Read the model definition and answer for the solid it produces. Units are mm, in the model's axes. A direction names the side the tool comes from. Coordinates: 2 decimals unless noted, no trailing zeros.
Item 1: A tool of negligible diameter and unlimited length cuts with its end or side. For faces 1 (the face through (3.035, 15.486, 2.465)), 2 (the face through (-3.035, -15.486, 2.465)), 3 (the face through (-2, 9, 5)), 4 (the face through (-1.5, 11.4, -1)), from which of +Z, -Z, +X, -X, +Y, -Y can it reach the whole face along a straight path? Write none if from no direction.
Item 2: Each of these flat-tipped pins is pushed along its axis until it touches: P1, Ø1.5, axis at x = 2, z = 1.5, coming from the +Y side; P2, Ø20.5, axis at x = 0, y = 0, coming from the +Z side; P3, Ø5, axis at y = 8, z = 3.5, coming from the +X side; P4, Ø11.5, axis at x = -0.5, y = 2, coming from the -Z side. Where does it stop, or does it pass through?
Item 3: Straight lines are drawn through the part: probe 1 along Y at (x, z) = (0, 5.75); probe 2 along Z at (x, y) = (-10.5, -10); probe 3 along X at (y, z) = (1.5, 3.25). For each, find the intervals that lie inside material, in ascending order.
Item 4: Determine the mould class of faces 5 (the face through (-13.84, 7.99, 2.46)), 6 (the face through (5.465, -15.015, 2.465)), 7 (the face through (15.736, -2.775, 2.465)), 8 (the face through (-2, 9, 0)) for opening direction Y: released by +Y, released by -Y, zero draft, split by the parting line, or undercut.
from build123d import *

# Parameters (mm, degrees)
F1_DEPTH = 5
F2_R     = 13.25
F2_R_2   = 11.5
F3_DEPTH = 2.5
F4_R     = 13.25
F4_R_2   = 11.5
F5_DEPTH = 2.5
F6_R     = 0.5


with BuildPart() as f1:
    # F0 (on Top) → F1 (new body)
    with BuildSketch(Plane.XY):
        with BuildLine():
            Line((3.0937469913, 8.5), (4.9592920782, 13.6255430014))
            ThreePointArc((4.9592920782, 13.6255430014), (2.5178985762, 14.2797124187), (0, 14.5))
            Line((0, 14.5), (0, 8.5))
            Line((0, 8.5), (3.0937469913, 8.5))
        make_face()
        with BuildLine():
            ThreePointArc((0, 14.5), (2.5178985762, 14.2797124187), (4.9592920782, 13.6255430014))
            Line((4.9592920782, 13.6255430014), (5.9853525082, 16.4446208638))
            Line((5.9853525082, 16.4446208638), (0, 14.5))
        make_face()
        with BuildLine():
            Line((-3.0937469913, 8.5), (0, 8.5))
            Line((0, 8.5), (0, 14.5))
            ThreePointArc((0, 14.5), (-2.5178985762, 14.2797124187), (-4.9592920782, 13.6255430014))
            Line((-4.9592920782, 13.6255430014), (-3.0937469913, 8.5))
        make_face()
        with BuildLine():
            ThreePointArc((-4.9592920782, 13.6255430014), (-2.5178985762, 14.2797124187), (0, 14.5))
            Line((0, 14.5), (0, 17.5))
            Line((0, 17.5), (-4.9592920782, 13.6255430014))
        make_face()
        with BuildLine():
            Line((5.8143424365, 6.9292634873), (9.3204203405, 11.1076444252))
            ThreePointArc((9.3204203405, 11.1076444252), (7.25, 12.5573683549), (4.9592920782, 13.6255430014))
            Line((4.9592920782, 13.6255430014), (3.0937469913, 8.5))
            Line((3.0937469913, 8.5), (4.9074772881, 8.5))
            Line((4.9074772881, 8.5), (5.8143424365, 6.9292634873))
        make_face()
        with BuildLine():
            ThreePointArc((4.9592920782, 13.6255430014), (7.25, 12.5573683549), (9.3204203405, 11.1076444252))
            Line((9.3204203405, 11.1076444252), (11.2487831695, 13.4057777546))
            Line((11.2487831695, 13.4057777546), (4.9592920782, 13.6255430014))
        make_face()
        with BuildLine():
            ThreePointArc((9.3204203405, 11.1076444252), (11.1076444252, 9.3204203405), (12.5573683549, 7.25))
            Line((12.5573683549, 7.25), (15.1554445662, 8.75))
            Line((15.1554445662, 8.75), (9.3204203405, 11.1076444252))
        make_face()
        with BuildLine():
            Line((8.9080894278, 1.5707365127), (14.2797124187, 2.5178985762))
            ThreePointArc((14.2797124187, 2.5178985762), (13.6255430014, 4.9592920782), (12.5573683549, 7.25))
            Line((12.5573683549, 7.25), (7.3612159322, 4.25))
            Line((7.3612159322, 4.25), (8.9080894278, 1.5707365127))
        make_face()
        with BuildLine():
            ThreePointArc((12.5573683549, 7.25), (13.6255430014, 4.9592920782), (14.2797124187, 2.5178985762))
            Line((14.2797124187, 2.5178985762), (17.2341356777, 3.0388431092))
            Line((17.2341356777, 3.0388431092), (12.5573683549, 7.25))
        make_face()
        with BuildLine():
            ThreePointArc((14.2797124187, -2.5178985762), (14.4448231223, -1.2637582698), (14.5, 0))
            ThreePointArc((14.5, 0), (14.4448231223, 1.2637582698), (14.2797124187, 2.5178985762))
            Line((14.2797124187, 2.5178985762), (8.9080894278, 1.5707365127))
            Line((8.9080894278, 1.5707365127), (9.8149545762, 0))
            Line((9.8149545762, 0), (8.9080894278, -1.5707365127))
            Line((8.9080894278, -1.5707365127), (14.2797124187, -2.5178985762))
        make_face()
        with BuildLine():
            ThreePointArc((14.2797124187, 2.5178985762), (14.4448231223, 1.2637582698), (14.5, 0))
            ThreePointArc((14.5, 0), (14.4448231223, -1.2637582698), (14.2797124187, -2.5178985762))
            Line((14.2797124187, -2.5178985762), (17.2341356777, -3.0388431092))
            Line((17.2341356777, -3.0388431092), (14.2797124187, 2.5178985762))
        make_face()
        with BuildLine():
            ThreePointArc((12.5573683549, -7.25), (13.6255430014, -4.9592920782), (14.2797124187, -2.5178985762))
            Line((14.2797124187, -2.5178985762), (8.9080894278, -1.5707365127))
            Line((8.9080894278, -1.5707365127), (7.3612159322, -4.25))
            Line((7.3612159322, -4.25), (12.5573683549, -7.25))
        make_face()
        with BuildLine():
            Line((15.1554445662, -8.75), (14.2797124187, -2.5178985762))
            ThreePointArc((14.2797124187, -2.5178985762), (13.6255430014, -4.9592920782), (12.5573683549, -7.25))
            Line((12.5573683549, -7.25), (15.1554445662, -8.75))
        make_face()
        with BuildLine():
            ThreePointArc((9.3204203405, -11.1076444252), (11.1076444252, -9.3204203405), (12.5573683549, -7.25))
            Line((12.5573683549, -7.25), (7.3612159322, -4.25))
            Line((7.3612159322, -4.25), (5.8143424365, -6.9292634873))
            Line((5.8143424365, -6.9292634873), (9.3204203405, -11.1076444252))
        make_face()
        with BuildLine():
            Line((11.2487831695, -13.4057777546), (12.5573683549, -7.25))
            ThreePointArc((12.5573683549, -7.25), (11.1076444252, -9.3204203405), (9.3204203405, -11.1076444252))
            Line((9.3204203405, -11.1076444252), (11.2487831695, -13.4057777546))
        make_face()
        with BuildLine():
            ThreePointArc((4.9592920782, -13.6255430014), (7.25, -12.5573683549), (9.3204203405, -11.1076444252))
            Line((9.3204203405, -11.1076444252), (5.8143424365, -6.9292634873))
            Line((5.8143424365, -6.9292634873), (4.9074772881, -8.5))
            Line((4.9074772881, -8.5), (3.0937469913, -8.5))
            Line((3.0937469913, -8.5), (4.9592920782, -13.6255430014))
        make_face()
        with BuildLine():
            Line((5.9853525082, -16.4446208638), (9.3204203405, -11.1076444252))
            ThreePointArc((9.3204203405, -11.1076444252), (7.25, -12.5573683549), (4.9592920782, -13.6255430014))
            Line((4.9592920782, -13.6255430014), (5.9853525082, -16.4446208638))
        make_face()
        with BuildLine():
            Line((0, -17.5), (4.9592920782, -13.6255430014))
            ThreePointArc((4.9592920782, -13.6255430014), (2.5178985762, -14.2797124187), (0, -14.5))
            Line((0, -14.5), (0, -17.5))
        make_face()
        with BuildLine():
            Line((0, -8.5), (-3.0937469913, -8.5))
            Line((-3.0937469913, -8.5), (-4.9592920782, -13.6255430014))
            ThreePointArc((-4.9592920782, -13.6255430014), (-2.5178985762, -14.2797124187), (0, -14.5))
            Line((0, -14.5), (0, -8.5))
        make_face()
        with BuildLine():
            ThreePointArc((0, -14.5), (-2.5178985762, -14.2797124187), (-4.9592920782, -13.6255430014))
            Line((-4.9592920782, -13.6255430014), (-5.9853525082, -16.4446208638))
            Line((-5.9853525082, -16.4446208638), (0, -14.5))
        make_face()
        with BuildLine():
            Line((7.3612159322, 4.25), (12.5573683549, 7.25))
            ThreePointArc((12.5573683549, 7.25), (11.1076444252, 9.3204203405), (9.3204203405, 11.1076444252))
            Line((9.3204203405, 11.1076444252), (5.8143424365, 6.9292634873))
            Line((5.8143424365, 6.9292634873), (7.3612159322, 4.25))
        make_face()
        with BuildLine():
            Line((3.0937469913, -8.5), (0, -8.5))
            Line((0, -8.5), (0, -14.5))
            ThreePointArc((0, -14.5), (2.5178985762, -14.2797124187), (4.9592920782, -13.6255430014))
            Line((4.9592920782, -13.6255430014), (3.0937469913, -8.5))
        make_face()
        with BuildLine():
            Line((-4.9074772881, -8.5), (-5.8143424365, -6.9292634873))
            Line((-5.8143424365, -6.9292634873), (-9.3204203405, -11.1076444252))
            ThreePointArc((-9.3204203405, -11.1076444252), (-7.25, -12.5573683549), (-4.9592920782, -13.6255430014))
            Line((-4.9592920782, -13.6255430014), (-3.0937469913, -8.5))
            Line((-3.0937469913, -8.5), (-4.9074772881, -8.5))
        make_face()
        with BuildLine():
            ThreePointArc((-4.9592920782, -13.6255430014), (-7.25, -12.5573683549), (-9.3204203405, -11.1076444252))
            Line((-9.3204203405, -11.1076444252), (-11.2487831695, -13.4057777546))
            Line((-11.2487831695, -13.4057777546), (-4.9592920782, -13.6255430014))
        make_face()
        with BuildLine():
            ThreePointArc((-9.3204203405, -11.1076444252), (-11.1076444252, -9.3204203405), (-12.5573683549, -7.25))
            Line((-12.5573683549, -7.25), (-15.1554445662, -8.75))
            Line((-15.1554445662, -8.75), (-9.3204203405, -11.1076444252))
        make_face()
        with BuildLine():
            Line((-5.8143424365, -6.9292634873), (-7.3612159322, -4.25))
            Line((-7.3612159322, -4.25), (-12.5573683549, -7.25))
            ThreePointArc((-12.5573683549, -7.25), (-11.1076444252, -9.3204203405), (-9.3204203405, -11.1076444252))
            Line((-9.3204203405, -11.1076444252), (-5.8143424365, -6.9292634873))
        make_face()
        with BuildLine():
            ThreePointArc((-12.5573683549, -7.25), (-13.6255430014, -4.9592920782), (-14.2797124187, -2.5178985762))
            Line((-14.2797124187, -2.5178985762), (-17.2341356777, -3.0388431092))
            Line((-17.2341356777, -3.0388431092), (-12.5573683549, -7.25))
        make_face()
        with BuildLine():
            Line((-7.3612159322, -4.25), (-8.9080894278, -1.5707365127))
            Line((-8.9080894278, -1.5707365127), (-14.2797124187, -2.5178985762))
            ThreePointArc((-14.2797124187, -2.5178985762), (-13.6255430014, -4.9592920782), (-12.5573683549, -7.25))
            Line((-12.5573683549, -7.25), (-7.3612159322, -4.25))
        make_face()
        with BuildLine():
            ThreePointArc((-14.2797124187, -2.5178985762), (-14.5, 0), (-14.2797124187, 2.5178985762))
            Line((-14.2797124187, 2.5178985762), (-17.2341356777, 3.0388431092))
            Line((-17.2341356777, 3.0388431092), (-14.2797124187, -2.5178985762))
        make_face()
        with BuildLine():
            Line((-9.8149545762, 0), (-8.9080894278, 1.5707365127))
            Line((-8.9080894278, 1.5707365127), (-14.2797124187, 2.5178985762))
            ThreePointArc((-14.2797124187, 2.5178985762), (-14.5, 0), (-14.2797124187, -2.5178985762))
            Line((-14.2797124187, -2.5178985762), (-8.9080894278, -1.5707365127))
            Line((-8.9080894278, -1.5707365127), (-9.8149545762, 0))
        make_face()
        with BuildLine():
            ThreePointArc((-14.2797124187, 2.5178985762), (-13.6255430014, 4.9592920782), (-12.5573683549, 7.25))
            Line((-12.5573683549, 7.25), (-15.1554445662, 8.75))
            Line((-15.1554445662, 8.75), (-14.2797124187, 2.5178985762))
        make_face()
        with BuildLine():
            Line((-8.9080894278, 1.5707365127), (-7.3612159322, 4.25))
            Line((-7.3612159322, 4.25), (-12.5573683549, 7.25))
            ThreePointArc((-12.5573683549, 7.25), (-13.6255430014, 4.9592920782), (-14.2797124187, 2.5178985762))
            Line((-14.2797124187, 2.5178985762), (-8.9080894278, 1.5707365127))
        make_face()
        with BuildLine():
            ThreePointArc((-12.5573683549, 7.25), (-11.1076444252, 9.3204203405), (-9.3204203405, 11.1076444252))
            Line((-9.3204203405, 11.1076444252), (-11.2487831695, 13.4057777546))
            Line((-11.2487831695, 13.4057777546), (-12.5573683549, 7.25))
        make_face()
        with BuildLine():
            Line((-7.3612159322, 4.25), (-5.8143424365, 6.9292634873))
            Line((-5.8143424365, 6.9292634873), (-9.3204203405, 11.1076444252))
            ThreePointArc((-9.3204203405, 11.1076444252), (-11.1076444252, 9.3204203405), (-12.5573683549, 7.25))
            Line((-12.5573683549, 7.25), (-7.3612159322, 4.25))
        make_face()
        with BuildLine():
            ThreePointArc((-9.3204203405, 11.1076444252), (-7.25, 12.5573683549), (-4.9592920782, 13.6255430014))
            Line((-4.9592920782, 13.6255430014), (-5.9853525082, 16.4446208638))
            Line((-5.9853525082, 16.4446208638), (-9.3204203405, 11.1076444252))
        make_face()
        with BuildLine():
            Line((-4.9074772881, 8.5), (-3.0937469913, 8.5))
            Line((-3.0937469913, 8.5), (-4.9592920782, 13.6255430014))
            ThreePointArc((-4.9592920782, 13.6255430014), (-7.25, 12.5573683549), (-9.3204203405, 11.1076444252))
            Line((-9.3204203405, 11.1076444252), (-5.8143424365, 6.9292634873))
            Line((-5.8143424365, 6.9292634873), (-4.9074772881, 8.5))
        make_face()
    extrude(amount=F1_DEPTH)

    # F2 (on face) → F3 (join)
    with BuildSketch(Plane.XY.offset(5)):
        Circle(F2_R)
        Circle(F2_R_2, mode=Mode.SUBTRACT)
    extrude(amount=F3_DEPTH)

    # F4 (on face) → F5 (join)
    with BuildSketch(Plane.XY):
        Circle(F4_R)
        Circle(F4_R_2, mode=Mode.SUBTRACT)
    extrude(amount=-F5_DEPTH)

    # F6
    f6_edges = [f1.edges().sort_by_distance(p)[0] for p in [
        (-13.25, 0, 7.5),
        (-11.5, 0, 7.5),
        (-13.25, 0, -2.5),
        (-11.5, 0, -2.5),
    ]]
    fillet(f6_edges, radius=F6_R)


solid = f1.part
Established:
1. face 1: +Z, -Z, +Y
1. face 2: +Z, -Z, -Y
1. face 3: +Z
1. face 4: -Z
2. P1: stops at y = 15.39
2. P2: stops at z = 5
2. P3: stops at x = 15.16
2. P4: passes through
3. probe 1: y = -13.25 to -11.5, 11.5 to 13.25
3. probe 2: z = 0 to 5
3. probe 3: x = -16.42 to -8.95, 8.95 to 14.82
4. face 5: released by +Y
4. face 6: released by -Y
4. face 7: undercut
4. face 8: undercut
